Autodesk Inventor part; units mm, degrees
ref_plane "YZ Plane" through (0, 0, 0) normal (1, 0, 0) x (0, 1, 0)
ref_plane "XZ Plane" through (0, 0, 0) normal (0, 1, 0) x (-1, 0, 0)
ref_plane "XY Plane" through (0, 0, 0) normal (0, 0, 1) x (1, 0, 0)
sketch "Sketch1" plane through (0, 0, 0) normal (0, 1, 0) x (-1, 0, 0)
  circle A0 centre (0, 0) radius 5.5
  dimension "d0" = 11
extrude "Extrusion1" add sketch "Sketch1" along normal blind 8
sketch "Sketch2" plane through (0, 0, 0) normal (1, 0, 0) x (0, 1, 0)
  line L0 (0, 0) -> (2.7456, 0)
  line L1 (2.25, 0) -> (2.25, 3.375)
  line L2 (2.25, 3.375) -> (0, 2.076)
  line L3 (0, -5.5) -> (0, 5.5) construction
  line L4 (2.25, 0) -> (2.25, -3.375)
  line L5 (2.25, -3.375) -> (0, -2.076)
  line L6 (0, -2.076) -> (0, 2.076)
  dimension "d9" = 3.375
  dimension "d10" = 2.25
  dimension "d11" = 60
extrude "Extrusion2" cut sketch "Sketch2" along normal through all both and the other way through all
sketch "Sketch3" plane through (0, 8, 0) normal (0, 1, 0) x (1, 0, 0)
  circle A0 centre (0, 0) radius 5.5
  line L0 (1.9486, 3.375) -> (3.8971, 0)
  line L1 (3.8971, 0) -> (1.9486, -3.375)
  line L2 (1.9486, -3.375) -> (-1.9486, -3.375)
  line L3 (-1.9486, -3.375) -> (-3.8971, 0)
  line L4 (-3.8971, 0) -> (-1.9486, 3.375)
  line L5 (-1.9486, 3.375) -> (1.9486, 3.375)
  circle A1 centre (0, 0) radius 2.625
  dimension "d14" = 6.75
  dimension "d15" = 5.25
extrude "Extrusion3" cut sketch "Sketch3" against normal blind 2.5 contours A1
extrude "Extrusion4" add sketch "Sketch3" along normal blind 14 contours A0
properties part number "Varf Biti"
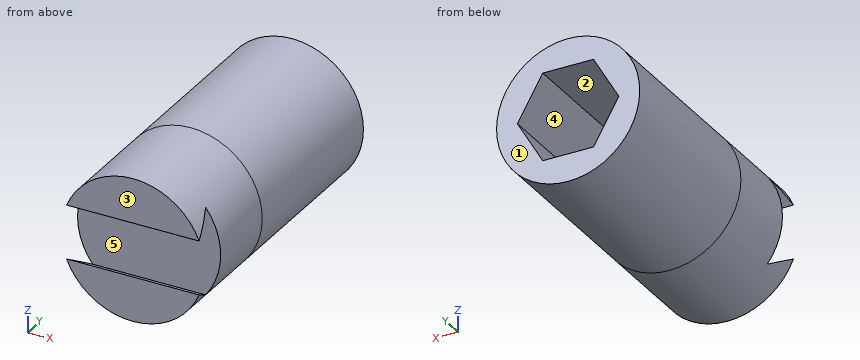
Could you check a few things on this model? Use its own coordinates, in mm. Face numbers are marked on the shaded views. A direction names the side the tool comes from. Coordinates: 2 decimals unless noted, no trailing zeros. Write each loop counter-clockwise with the first axis right and the second up, starting at its lowest first coordinate (ties: lowest second). Pieces come first, ordered by that corner, then holes. Notation, with made-up numbers: M 16.25,49 L 31.25,49 A16 cw 31.25,71 Z; hole C -3,6.25 d2. An arc over 180 degrees is marked long. Answer as CSV lines item,"result". Start each with the question number.
1) I want a section at D-D, the plane y = 7. Please give me the cut outline in (x, z) (3 decimals).
2) I want a section at A-A, the plane y = 17. Please give me the cut outline in (x, z) (3 decimals), and give its area (3 significant figures).
3) I want a section at C-C, the plane x = 0. Please give me the cut outline in (y, z) (3 decimals).
4) I want a section at B-B, the plane z = -3. Please give me the cut outline in (x, y).
5) For P1, Ø1, axis at x = -2.5, y = 11.5, coming from the -Z side; P2, Ø1.5, axis at x = -4, y = 18, coming from the +Z side; P3, Ø2, axis at x = 1.5, z = 0, coming from the +Y side, each with a flat end and sliding along its axis, tell me the tip position at first contact or that it passes through.
6) For the marked faces 3, 4 and 5, which set-ups out of +Z, -Z, +X, -X, +Y, -Y let a thin tool reach every point of the face, with its end or its side?
7) We'd pull the mould along X, two halves only. Please class the marked faces 1 and 2: +X half, -X half, draft (parallel to the pull), parting line (faces both ways), or undercut.
8) Please list where these lines run through material, in increasing order: line 1 (Z direction, x = 0, y = 7.55) (3 decimals); line 2 (Y direction, x = 2.5, z = -2.75). Write a range as from..to.
Data:
1,outline,"C 0,0 d11; hole C 0,0 d5.25"
2,outline,"C 0,0 d11; hole M -3.897,0 L -1.949,-3.375 L 1.949,-3.375 L 3.897,0 L 1.949,3.375 L -1.949,3.375 Z"
2,area,"55.6 mm^2"
3,outline,"M 0,-5.5 L 22,-5.5 L 22,-3.375 L 8,-3.375 L 8,-2.625 L 5.5,-2.625 L 5.5,2.625 L 8,2.625 L 8,3.375 L 22,3.375 L 22,5.5 L 0,5.5 L 0,2.076 L 2.25,3.375 L 2.25,-3.375 L 0,-2.076 Z"
4,outline,"M -4.61,0 L 4.61,0 L 4.61,1.6 L -4.61,1.6 Z; M -4.61,2.25 L 4.61,2.25 L 4.61,22 L 2.17,22 L 2.17,8 L -2.17,8 L -2.17,22 L -4.61,22 Z"
5,P1,"stops at z = -5.12"
5,P2,"stops at z = 4.44"
5,P3,"stops at y = 5.5"
6,face 3,"+Z, -Z, +X, -X, -Y"
6,face 4,"+Y"
6,face 5,"+X, -X"
7,face 1,"draft"
7,face 2,"undercut"
8,line 1,"z = -5.5..-2.625, 2.625..5.5"
8,line 2,"y = 0..1.17, 2.25..22"
